Here's how the part is built. I have some questions about the finished solid (model axes, mm). A direction names the side the tool comes from. Coordinates: 2 decimals unless noted, no trailing zeros. Loops run counter-clockwise (first coordinate to the right, second up) from the corner with the lowest first, then second, coordinate; pieces in that order, holes last.
```python
from build123d import *

# Parameters (mm, degrees)
EXTRUDE_1_DEPTH        = 10
SKETCH_2_R             = 0.95
CUT_EXTRUDE_1_DEPTH    = 5
FILLET_1_R             = 3
CHAMFER_2_SIZE         = 1
EXTRUDE_START          = 1.5
EXTRUDE_2_DEPTH        = 1.5
FILLET_2_R             = 3
SKETCH_5_W             = 18.894194267
SKETCH_5_H             = 13.568314004
CUT_EXTRUDE_1877_DEPTH = 10.5


with BuildPart() as part:
    # 草图1 → 凸台-拉伸1 (new body)
    with BuildSketch(Plane.XY):
        Polygon((0, 0), (18, 0), (18, -7.86), (14, -7.86), (14, -3), (1, -3), (1, -7.86), (-3, -7.86), (-3, 12), (0, 12), align=None)
    extrude(amount=EXTRUDE_1_DEPTH)

    # 草图2 → 切除-拉伸1 (cut)
    with BuildSketch(Plane.XZ.offset(7.86)):
        with Locations((-1, 5)):
            Circle(SKETCH_2_R)
        with Locations((16, 5.10136652)):
            Circle(SKETCH_2_R)
    extrude(amount=-CUT_EXTRUDE_1_DEPTH, mode=Mode.SUBTRACT)

    # 圆角1
    fillet_1_edges = [part.edges().sort_by_distance(p)[0] for p in [
        (14, -3, 5),
        (1, -3, 5),
    ]]
    fillet(fillet_1_edges, radius=FILLET_1_R)

    # 倒角2
    chamfer_2_edges = [part.edges().sort_by_distance(p)[0] for p in [
        (-1.95, -7.86, 5),
        (15.05, -7.86, 5.10136652),
    ]]
    chamfer(chamfer_2_edges, length=CHAMFER_2_SIZE)

    # 草图4 → 凸台-拉伸2 (add)
    with BuildSketch(Plane.XY.offset(10).offset(EXTRUDE_START)):
        with BuildLine():
            Line((0, 12), (0, 3))
            Line((0, 3), (18, 3))
            Line((18, 3), (18, 0))
            Line((18, 0), (18, -7.86))
            Line((18, -7.86), (14, -7.86))
            Line((14, -7.86), (14, -6))
            ThreePointArc((14, -6), (13.121320344, -3.878679656), (11, -3))
            Line((11, -3), (4, -3))
            ThreePointArc((4, -3), (1.878679656, -3.878679656), (1, -6))
            Line((1, -6), (1, -7.86))
            Line((1, -7.86), (-3, -7.86))
            Line((-3, -7.86), (-3, 12))
            Line((-3, 12), (0, 12))
        make_face()
    extrude(amount=-EXTRUDE_2_DEPTH)

    # 圆角2
    fillet_2_edges = [part.edges().sort_by_distance(p)[0] for p in [
        (0, 3, 10.75),
    ]]
    fillet(fillet_2_edges, radius=FILLET_2_R)

    # 草图5 → Cut-Extrude 1877 (cut)
    with BuildSketch(Plane(origin=(0, 0, 0), x_dir=(-1, 0, 0), z_dir=(0, 0, -1))):
        with Locations((-8.947097133, 6.284157002)):
            Rectangle(SKETCH_5_W, SKETCH_5_H)
    extrude(amount=-CUT_EXTRUDE_1877_DEPTH, mode=Mode.SUBTRACT)


solid = part.part
```
1. I want a section at D-D (x = 16). Please give me the cut outline in (y, z).
2. For pin 1 (1.7 mm diameter, centred on x = -1, z = 5, fed in from -Y); pin 2 (4 mm diameter, centred on y = 7.5, z = 6.5, fed in from +X); pin 3 (1.1 mm diameter, centred on x = 16, z = 5.1, fed in from +Y), each with a flat end and sliding along its axis, tell me the tip position at first contact or that it passes through.
3. I need wall thicknesses on line 1 along Y through (x, z) = (10.75, 3.25); line 2 along Y through (x, z) = (16.75, 11.25). Which ranges of each line are inside material? Lowest first, please.
4. I want a section at A-A (y = -4.5). Please give me the cut outline in (x, z).
5. I want a section at C-C (y = 8.5). Please give me the cut outline in (x, z).
6. On a 3-axis mill with a long thin cutter (end or side, diameter ignored), from which of +Z, -Z, +X, -X, +Y, -Y can I reach the whole of each face in a straight line? I mean faces 5 (the flat face through (14, -7, 6)), 6 (the flat face through (18, -4, 6)), 7 (the flat face through (8, 2, 10.5)), 8 (the flat face through (-0.97, -7.86, 7.11)), 9 (the cylindrical face through (-0.56, -4.89, 4.16)). Say none if no direction works.
7. We'd pull the mould along Z, two halves only. Please class faces 1 (the flat face through (5, -1, 0)), 2 (the flat face through (-1, -2.86, 5)), 3 (the flat face through (0, 9, 11)), 4 (the flat face through (8, 0, 11.5)): +Z half, -Z half, draft (parallel to the pull), parting line (faces both ways), or undercut.
8. I want a section at B-B (x = -1). Please give me the cut outline in (y, z), then the cut area to 3 significant figures.
Response values:
1. outline: (-7.86, 0) - (-0.5, 0) - (-0.5, 10.5) - (3, 10.5) - (3, 11.5) - (-7.86, 11.5) - (-7.86, 7.05) - (-6.86, 6.05) - (-2.86, 6.05) - (-2.86, 4.15) - (-6.86, 4.15) - (-7.86, 3.15) - close
2. pin 1: stops at y = -2.86
2. pin 2: stops at x = -0.5
2. pin 3: stops at y = -0.5
3. line 1: y = -3 to -0.5
3. line 2: y = -7.86 to 3
4. outline: (-3, 0) - (1.4, 0) - (1.4, 11.5) - (-3, 11.5) - close; (13.6, 0) - (18, 0) - (18, 11.5) - (13.6, 11.5) - close; hole circle Ø1.9 at (-1, 5); hole circle Ø1.9 at (16, 5.1)
5. outline: (-3, 0) - (-0.5, 0) - (-0.5, 10.5) - (0, 10.5) - (0, 11.5) - (-3, 11.5) - close
6. face 5: +Z, -Z, -Y
6. face 6: +Z, -Z, +X, +Y, -Y
6. face 7: -Z, +X, +Y
6. face 8: +Z, -Z, +X, -X, -Y
6. face 9: -Y
7. face 1: -Z half
7. face 2: undercut
7. face 3: draft
7. face 4: +Z half
8. outline: (-7.86, 0) - (12, 0) - (12, 11.5) - (-7.86, 11.5) - (-7.86, 6.95) - (-6.86, 5.95) - (-2.86, 5.95) - (-2.86, 4.05) - (-6.86, 4.05) - (-7.86, 3.05) - close
8. area: 218 mm2
